```python
from build123d import *

# Parameters (mm, degrees)
SKETCH1_R           = 12.5
BOSS_EXTRUDE1_DEPTH = 7.5
SKETCH2_W           = 35
SKETCH2_H           = 8.580767914
BOSS_EXTRUDE2_DEPTH = 25
SKETCH3_W           = 25
SKETCH3_H           = 8.580767914
CUT_EXTRUDE1_DEPTH  = 20
SKETCH4_R           = 2.5
BOSS_EXTRUDE3_DEPTH = 6.25
SKETCH5_R           = 2.5
BOSS_EXTRUDE4_DEPTH = 6.25
CHAMFER1_SIZE       = 5
CHAMFER2_SIZE       = 5


with BuildPart() as part:
    # Sketch1 → Boss-Extrude1 (new body)
    with BuildSketch(Plane(origin=(0, 0, 0), x_dir=(1, 0, 0), z_dir=(0, 1, 0))):
        Circle(SKETCH1_R)
    extrude(amount=BOSS_EXTRUDE1_DEPTH)

    # Sketch2 → Boss-Extrude2 (add)
    with BuildSketch(Plane(origin=(0, 7.5, 0), x_dir=(1, 0, 0), z_dir=(0, 1, 0))):
        Rectangle(SKETCH2_W, SKETCH2_H)
    extrude(amount=BOSS_EXTRUDE2_DEPTH)

    # Sketch3 → Cut-Extrude1 (cut)
    with BuildSketch(Plane(origin=(0, 32.5, 0), x_dir=(1, 0, 0), z_dir=(0, 1, 0))):
        Rectangle(SKETCH3_W, SKETCH3_H)
    extrude(amount=-CUT_EXTRUDE1_DEPTH, mode=Mode.SUBTRACT)

    # Sketch4 → Boss-Extrude3 (add)
    with BuildSketch(Plane(origin=(-12.5, 0, 0), x_dir=(0, 0, -1), z_dir=(1, 0, 0))):
        with Locations((0, 27.5)):
            Circle(SKETCH4_R)
    extrude(amount=BOSS_EXTRUDE3_DEPTH)

    # Sketch5 → Boss-Extrude4 (add)
    with BuildSketch(Plane.ZY.offset(-12.5)):
        with Locations((0, 27.5)):
            Circle(SKETCH5_R)
    extrude(amount=BOSS_EXTRUDE4_DEPTH)

    # Chamfer1
    chamfer1_edges = [part.edges().sort_by_distance(p)[0] for p in [
        (-12.5, 12.5, 0),
    ]]
    chamfer(chamfer1_edges, length=CHAMFER1_SIZE)

    # Chamfer2
    chamfer2_edges = [part.edges().sort_by_distance(p)[0] for p in [
        (12.5, 12.5, 0),
    ]]
    chamfer(chamfer2_edges, length=CHAMFER2_SIZE)


solid = part.part
```
Read the model definition and answer for the solid it produces. Units are mm, in the model's axes. A direction names the side the tool comes from. Round coordinates to 2 decimals unless told otherwise and drop trailing zeros. Write each loop counter-clockwise with the first axis right and the second up, starting at its lowest first coordinate (ties: lowest second). Pieces come first, ordered by that corner, then holes. Notation, with made-up numbers: (-37.75, -24.75) -> (19.25, -24.75) arc R18 cw to (19.25, -6.75) -> close; hole circle Ø1 at (-11, -5). An arc over 180 degrees is marked (long way). Answer in a Markdown table with one row per item. Add a question column.
1) Find section B-B, the plane z = 0. Determine the outline of the cut face in (x, y).
2) Find section D-D, the plane y = 7. Determine the outline of the cut face in (x, z), and give its area (3 significant figures).
3) Given P1, Ø6.5, axis at x = -16, z = 1.5, coming from the -Y side; P2, Ø5, axis at x = -8, z = 7.5, coming from the +Y side; P3, Ø6, axis at x = -13, y = 4, coming from the +Z side; P4, Ø6, axis at y = 28, z = 9.5, coming from the -X side, each flat-ended and moving along its own axis, determine where each tip first touches the part or whether it passes through.
4) Which of the six approach directions +Z, -Z, +X, -X, +Y, -Y give full straight-line access (tool end or side, diameter ignored) to faces 5 (the face through (0, 11, -4.29)), 6 (the face through (0, 11, 4.29)), 7 (the face through (-6.25, 28, 0))?
5) Determine the mould class of faces 1 (the face through (11.923, 3.698, -3.755)), 2 (the face through (-10, 15, 0)), 3 (the face through (0, 0, 0)), 4 (the face through (6.25, 28, 0)) for opening direction X: pulls with the +X half, pulls with the -X half, needs draft (parallel to the pull), parting line crosses it, or undercut.
6) Find section A-A, the plane y = 27.5. Determine the outline of the cut face in (x, z).
7) Find section C-C, the plane x = 0. Determine the outline of the cut face in (y, z), and give its area (3 significant figures).
8) Consider line 1 (X direction, y = 19, z = 1); line 2 (Y direction, x = -4.5, z = 8.5); line 3 (Y direction, x = 2, z = 0). Determine where each line is inside the solid, lowest interval first.
Findings below:
| question | item | result |
|---|---|---|
| 1 | outline | (-17.5, 7.5) -> (-12.5, 7.5) -> (-12.5, 0) -> (12.5, 0) -> (12.5, 7.5) -> (17.5, 7.5) -> (17.5, 32.5) -> (12.5, 32.5) -> (12.5, 30) -> (6.25, 30) -> (6.25, 25) -> (12.5, 25) -> (12.5, 17.5) -> (7.5, 12.5) -> (-7.5, 12.5) -> (-12.5, 17.5) -> (-12.5, 25) -> (-6.25, 25) -> (-6.25, 30) -> (-12.5, 30) -> (-12.5, 32.5) -> (-17.5, 32.5) -> close |
| 2 | outline | circle Ø25 at (0, 0) |
| 2 | area | 491 mm² |
| 3 | P1 | y = 7.5 |
| 3 | P2 | y = 7.5 |
| 3 | P3 | z = 7.5 |
| 3 | P4 | through |
| 4 | face 5 | -Z, +X, -X, +Y |
| 4 | face 6 | +Z, +X, -X, +Y |
| 4 | face 7 | +Z, -Z, +Y |
| 5 | face 1 | parting line crosses it |
| 5 | face 2 | undercut |
| 5 | face 3 | needs draft |
| 5 | face 4 | undercut |
| 6 | outline | (-17.5, -4.29) -> (-12.5, -4.29) -> (-12.5, -2.5) -> (-6.25, -2.5) -> (-6.25, 2.5) -> (-12.5, 2.5) -> (-12.5, 4.29) -> (-17.5, 4.29) -> close; (6.25, -2.5) -> (12.5, -2.5) -> (12.5, -4.29) -> (17.5, -4.29) -> (17.5, 4.29) -> (12.5, 4.29) -> (12.5, 2.5) -> (6.25, 2.5) -> close |
| 7 | outline | (0, -12.5) -> (7.5, -12.5) -> (7.5, -4.29) -> (12.5, -4.29) -> (12.5, 4.29) -> (7.5, 4.29) -> (7.5, 12.5) -> (0, 12.5) -> close |
| 7 | area | 230 mm² |
| 8 | line 1 | -17.5 to -12.5, 12.5 to 17.5 |
| 8 | line 2 | 0 to 7.5 |
| 8 | line 3 | 0 to 12.5 |
